from build123d import *

# Parameters (mm, degrees)
SKETCH1_R           = 2.5
BOSS_EXTRUDE1_DEPTH = 5
SKETCH2_R           = 40
CUT_EXTRUDE1_DEPTH  = 2
CHAMFER1_SIZE       = 2.5


with BuildPart() as part:
    # Sketch1 → Boss-Extrude1 (new body)
    with BuildSketch(Plane(origin=(0, 0, 0), x_dir=(1, 0, 0), z_dir=(0, 1, 0))):
        with BuildLine():
            Line((-100, -53), (100, -53))
            ThreePointArc((100, -53), (153, 0), (100, 53))
            Line((100, 53), (-100, 53))
            ThreePointArc((-100, 53), (-153, 0), (-100, -53))
        make_face()
        with Locations((-100, -35)):
            Circle(SKETCH1_R, mode=Mode.SUBTRACT)
        with Locations((-100, 35)):
            Circle(SKETCH1_R, mode=Mode.SUBTRACT)
        with Locations((-69.689110868, 17.5)):
            Circle(SKETCH1_R, mode=Mode.SUBTRACT)
        with Locations((-69.689110868, -17.5)):
            Circle(SKETCH1_R, mode=Mode.SUBTRACT)
        with Locations((-130.310889132, 17.5)):
            Circle(SKETCH1_R, mode=Mode.SUBTRACT)
        with Locations((-130.310889132, -17.5)):
            Circle(SKETCH1_R, mode=Mode.SUBTRACT)
    extrude(amount=BOSS_EXTRUDE1_DEPTH)

    # Sketch2 → Cut-Extrude1 (cut)
    with BuildSketch(Plane(origin=(0, 5, 0), x_dir=(1, 0, 0), z_dir=(0, 1, 0))):
        with Locations((-100, 0)):
            Circle(SKETCH2_R)
    extrude(amount=-CUT_EXTRUDE1_DEPTH, mode=Mode.SUBTRACT)

    # Chamfer1
    chamfer1_edges = [part.edges().sort_by_distance(p)[0] for p in [
        (-153, 5, 0),
        (0, 5, 53),
        (153, 5, 0),
        (0, 5, -53),
    ]]
    chamfer(chamfer1_edges, length=CHAMFER1_SIZE)


solid = part.part
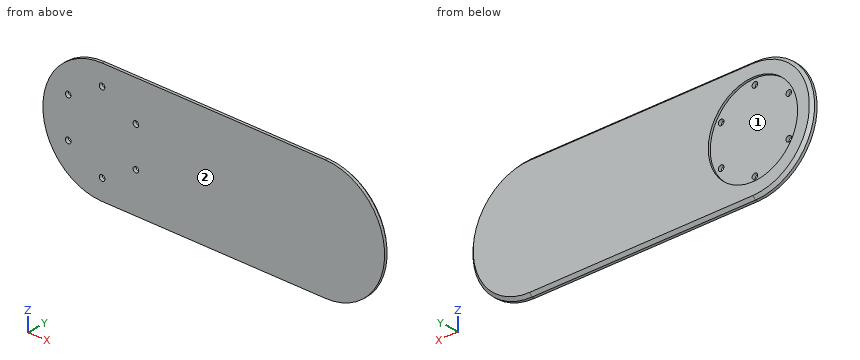
Model file for the job. Use its own axes, mm. Face numbers are marked on the shaded views. Coordinates: 2 decimals unless noted, no trailing zeros. Order: outer loops, then holes, each group sorted by start corner. A loop starts at its lowest first (then second) coordinate and runs counter-clockwise, first axis right, second up. Notation, with made-up numbers: (47, 20) -> (104, 20) arc R26 ccw to (104, 40) -> close; hole circle Ø4 at (13.25, -13). An arc over 180 degrees is marked (long way). Return JSON: item names as keys, results as strings. Group by question number.
Item 1: Saw through at B-B on z = 0. Write the cut outline in (x, y).
Item 2: Flat gauge pins, fed straight in: P1, Ø8, axis at x = -69.69, z = -17.5, coming from the +Y side; P2, Ø1.5, axis at x = -110, y = 3.5, coming from the +Z side; P3, Ø3, axis at x = -100, z = 35, coming from the +Y side (1 decimal); P4, Ø1.5, axis at x = 102.5, y = 3, coming from the -Z side. Where does each tip first touch, or does it go through?
Item 3: Saw through at A-A on y = 1.45. Write the cut outline in (x, z), then the cut area to 3 significant figures.
Item 4: Pull direction Z, two halves, no side cores. Call the marked faces 1 and 2: pulls with the +Z half, pulls with the -Z half, needs draft (parallel to the pull), parting line crosses it, or undercut.
Item 5: Wall check: line 1 along Z through (x, y) = (-100, 1.1); line 2 along X through (y, z) = (2.2, -17.5); line 3 along Z through (x, y) = (-101, 1.4). Give the ranges that are in metal, low to high. Write a range as [from, to].
Values found:
{
 "1": {"outline": "(-153, 0) -> (153, 0) -> (153, 2.5) -> (150.5, 5) -> (-60, 5) -> (-60, 3) -> (-140, 3) -> (-140, 5) -> (-150.5, 5) -> (-153, 2.5) -> close"},
 "2": {"P1": "stops at y = 3", "P2": "stops at z = 51.81", "P3": "passes through", "P4": "stops at z = -52.96"},
 "3": {"outline": "(-100, -53) -> (100, -53) arc R53 ccw to (100, 53) -> (-100, 53) arc R53 ccw to start; hole circle Ø5 at (-130.31, -17.5); hole circle Ø5 at (-130.31, 17.5); hole circle Ø5 at (-100, -35); hole circle Ø5 at (-100, 35); hole circle Ø5 at (-69.69, -17.5); hole circle Ø5 at (-69.69, 17.5)", "area": "29,900 mm2"},
 "4": {"face 1": "undercut", "face 2": "needs draft"},
 "5": {"line 1": "z = [-53, -37.5], [-32.5, 32.5], [37.5, 53]", "line 2": "x = [-150.03, -132.81], [-127.81, -72.19], [-67.19, 150.03]", "line 3": "z = [-52.99, -37.29], [-32.71, 32.71], [37.29, 52.99]"}
}
